```python
from build123d import *

# Parameters (mm, degrees)
F0_W     = 56
F0_H     = 32
F0_R     = 2.5
F0_R_2   = 12.5
F1_DEPTH = 18
F3_DEPTH = 10


with BuildPart() as f1:
    # F0 (on Top) → F1 (new body)
    with BuildSketch(Plane.XY):
        with Locations((0.009827, -16)):
            Rectangle(F0_W, F0_H)
        with Locations((-15.990173, -14)):
            Circle(F0_R, mode=Mode.SUBTRACT)
        with Locations((0.009827, -14)):
            Circle(F0_R_2, mode=Mode.SUBTRACT)
        with Locations((16.009827, -14)):
            Circle(F0_R, mode=Mode.SUBTRACT)
    extrude(amount=F1_DEPTH)

    # F2 (on face) → F3 (cut)
    with BuildSketch(Plane(origin=(0, 0, 0), x_dir=(-1, 0, 0), z_dir=(0, 1, 0))):
        with BuildLine():
            ThreePointArc((18.490173, 9), (20.990173, 6.5), (23.490173, 9))
            Line((23.490173, 9), (18.490173, 9))
        make_face()
        with BuildLine():
            Line((18.490173, 9), (23.490173, 9))
            ThreePointArc((23.490173, 9), (20.990173, 11.5), (18.490173, 9))
        make_face()
        with BuildLine():
            ThreePointArc((-23.509827, 9), (-21.009827, 6.5), (-18.509827, 9))
            Line((-18.509827, 9), (-23.509827, 9))
        make_face()
        with BuildLine():
            Line((-23.509827, 9), (-18.509827, 9))
            ThreePointArc((-18.509827, 9), (-21.009827, 11.5), (-23.509827, 9))
        make_face()
    extrude(amount=-F3_DEPTH, mode=Mode.SUBTRACT)


solid = f1.part
```
Check sheet for the modelled part. Datum: model origin and axes. Units: mm. A direction names the side the tool comes from. Round coordinates to 2 decimals unless told otherwise and drop trailing zeros. Loops run counter-clockwise (first coordinate to the right, second up) from the corner with the lowest first, then second, coordinate; pieces in that order, holes last. Notation, with made-up numbers: M 72.25,-32.75 L 112.25,-32.75 A38 cw 112.25,6.25 Z; hole C 84,56.5 d3. An arc over 180 degrees is marked long. Answer as a JSON object with one key per item and string values.
1. Mould release check, pull along Z, two halves, no side actions. Record for faces 3 (the flat face through (0, 0, 9)), 4 (the flat face through (-7, -26, 18)), 5 (the cylindrical face through (-20.45, -4.93, 6.56)), 6 (the flat face through (21, -10, 9)): pulls with the +Z half, pulls with the -Z half, needs draft (parallel to the pull), parting line crosses it, or undercut.
Reply:
{"face 3": "needs draft", "face 4": "pulls with the +Z half", "face 5": "undercut", "face 6": "undercut"}
2. Section check B-B (y = -14). Record the boundary of the cut face in (x, z).
Reply:
{"outline": "M -27.99,0 L -18.49,0 L -18.49,18 L -27.99,18 Z; M -13.49,0 L -12.49,0 L -12.49,18 L -13.49,18 Z; M 12.51,0 L 13.51,0 L 13.51,18 L 12.51,18 Z; M 18.51,0 L 28.01,0 L 28.01,18 L 18.51,18 Z"}
3. Gauge pin test, flat ends, axial feed: P1, Ø3, axis at x = -6, y = -22.5, coming from the -Z side; P2, Ø1.5, axis at x = 20.5, z = 9, coming from the +Y side. Record the tip position at first contact, or that the pin passes through.
Reply:
{"P1": "passes through", "P2": "stops at y = -10"}
4. Scan lines: line 1 (Y direction, x = 0.5, z = 11.25); line 2 (X direction, y = -12, z = 5.75); line 3 (X direction, y = -15.5, z = 9.75). Record each from-to range of solid material in increasing order.
Reply:
{"line 1": "y = -32 to -26.49, -1.51 to 0", "line 2": "x = -27.99 to -17.49, -14.49 to -12.33, 12.35 to 14.51, 17.51 to 28.01", "line 3": "x = -27.99 to -17.99, -13.99 to -12.4, 12.42 to 14.01, 18.01 to 28.01"}
5. Section check A-A (z = 13). Record the boundary of the cut face in (x, y).
Reply:
{"outline": "M -27.99,-32 L 28.01,-32 L 28.01,0 L -27.99,0 Z; hole C -15.99,-14 d5; hole C 0.01,-14 d25; hole C 16.01,-14 d5"}
6. Section check D-D (z = 9). Record the boundary of the cut face in (x, y), plus the area to 3 significant figures.
Reply:
{"outline": "M -27.99,-32 L 28.01,-32 L 28.01,0 L 23.51,0 L 23.51,-10 L 18.51,-10 L 18.51,0 L -18.49,0 L -18.49,-10 L -23.49,-10 L -23.49,0 L -27.99,0 Z; hole C -15.99,-14 d5; hole C 0.01,-14 d25; hole C 16.01,-14 d5", "area": "1,160 mm²"}
7. Section check C-C (x = 9). Record the boundary of the cut face in (y, z).
Reply:
{"outline": "M -32,0 L -22.68,0 L -22.68,18 L -32,18 Z; M -5.32,0 L 0,0 L 0,18 L -5.32,18 Z"}
8. Access from +Z, -Z, +X, -X, +Y, -Y to the whole of each face (thin tool, end or side, straight path). Record for faces 1 (the cylindrical face through (19.86, -4.93, 6.78)), 2 (the cylindrical face through (18.3, -15, 8.9)).
Reply:
{"face 1": "+Y", "face 2": "+Z, -Z"}
